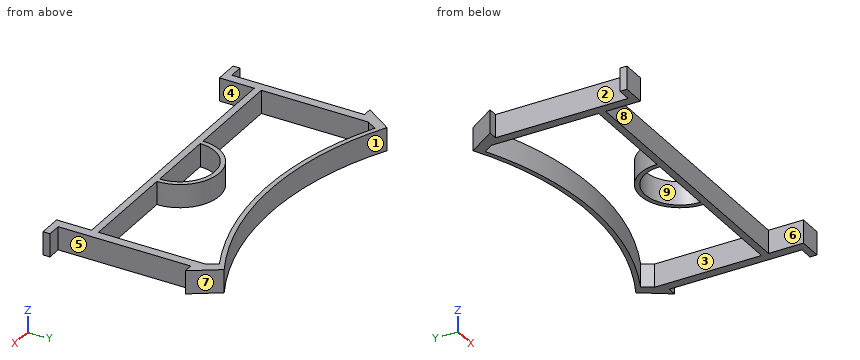
```python
from build123d import *

# Parameters (mm, degrees)
F1_DEPTH = 10


with BuildPart() as f1:
    # F0 (on Top) → F1 (new body)
    with BuildSketch(Plane.XY):
        with BuildLine():
            Line((0, 15), (0, 0))
            Line((0, 0), (10, 0))
            Line((10, 0), (10, 3))
            Line((10, 3), (4, 3))
            Line((4, 3), (4, 60))
            Line((4, 60), (8, 60))
            Line((8, 60), (0, 72))
            ThreePointArc((0, 72), (-60, 57.325626), (-120, 72))
            Line((-120, 72), (-128, 60))
            Line((-128, 60), (-124, 60))
            Line((-124, 60), (-124, 3))
            Line((-124, 3), (-130, 3))
            Line((-130, 3), (-130, 0))
            Line((-130, 0), (-120, 0))
            Line((-120, 0), (-120, 15))
            Line((-120, 15), (-120, 18))
            Line((-120, 18), (-120, 60))
            Line((-120, 60), (-120, 64))
            Line((-120, 64), (-117.309005, 68.39129))
            ThreePointArc((-117.309005, 68.39129), (-60, 55.232971), (-2.690995, 68.39129))
            Line((-2.690995, 68.39129), (0, 64))
            Line((0, 64), (0, 60))
            Line((0, 60), (0, 18))
            Line((0, 18), (0, 15))
        make_face()
        Polygon((-120, 15), (0, 15), (0, 18), (-43, 18), (-45, 18), (-75, 18), (-77, 18), (-120, 18), align=None)
        with BuildLine():
            Line((-45, 18), (-43, 18))
            ThreePointArc((-43, 18), (-60, 35), (-77, 18))
            Line((-77, 18), (-75, 18))
            ThreePointArc((-75, 18), (-60, 33), (-45, 18))
        make_face()
    extrude(amount=F1_DEPTH)


solid = f1.part
```
Verification items for the finished model (mm, model axes). Face numbers are marked on the shaded views. A direction names the side the tool comes from. Round coordinates to 2 decimals unless told otherwise and drop trailing zeros. Loops run counter-clockwise (first coordinate to the right, second up) from the corner with the lowest first, then second, coordinate; pieces in that order, holes last. Notation, with made-up numbers: (6.25, -34.5) -> (43.25, -34.5) arc R24 cw to (43.25, -4.5) -> close; hole circle Ø8 at (79, 15). An arc over 180 degrees is marked (long way). Answer as a JSON object with one key per item and string values.
Q1. Scan lines: line 1 (Y direction, x = -49, z = 3.25); line 2 (X direction, y = 10, z = 4.5); line 3 (Y direction, x = -68, z = 2). Record each from-to range of solid material in increasing order. Write a range as from..to.
Data:
{"line 1": "y = 15..18, 28.2..30.96, 55.69..57.79", "line 2": "x = -124..-120, 0..4", "line 3": "y = 15..18, 30.69..33, 55.48..57.57"}
Q2. Section check C-C (y = 50). Record the boundary of the cut face in (x, z).
Data:
{"outline": "(-124, 0) -> (-120, 0) -> (-120, 10) -> (-124, 10) -> close; (0, 0) -> (4, 0) -> (4, 10) -> (0, 10) -> close"}
Q3. Go/stop test with flat-tipped pins: P1, Ø3, axis at y = 40.5, z = 6.5, coming from the -X side; P2, Ø1.8, axis at x = 7.5, z = 5.5, coming from the +Y side; P3, Ø4, axis at y = 29.5, z = 2, coming from the +X side; P4, Ø10, axis at x = -85.5, y = 7.5, coming from the -Z side. Record where each tip stops, or that it passes through.
Data:
{"P1": "stops at x = -124", "P2": "stops at y = 62.1", "P3": "stops at x = 4", "P4": "passes through"}
Q4. Section check D-D (x = -31). Record the boundary of the cut face in (y, z), then the cut area to 3 significant figures.
Data:
{"outline": "(15, 0) -> (18, 0) -> (18, 10) -> (15, 10) -> close; (58.47, 0) -> (60.6, 0) -> (60.6, 10) -> (58.47, 10) -> close", "area": "51.3 mm2"}
Q5. Section check B-B (z = 2.25). Record the boundary of the cut face in (x, y), then the cut area to 3 significant figures.
Data:
{"outline": "(-130, 0) -> (-120, 0) -> (-120, 15) -> (0, 15) -> (0, 0) -> (10, 0) -> (10, 3) -> (4, 3) -> (4, 60) -> (8, 60) -> (0, 72) arc R130 cw to (-120, 72) -> (-128, 60) -> (-124, 60) -> (-124, 3) -> (-130, 3) -> close; hole (-120, 18) -> (-77, 18) arc R17 cw to (-43, 18) -> (0, 18) -> (0, 64) -> (-2.69, 68.39) arc R131.38 cw to (-117.31, 68.39) -> (-120, 64) -> close; hole (-75, 18) -> (-45, 18) arc R15 ccw to start", "area": "1,350 mm2"}
Q6. Draft check along Y on the marked faces 6, 7, 8 and 9. Enter one of: pulls with the +Y half, pulls with the -Y half, needs draft (parallel to the pull), parting line crosses it, or undercut.
Data:
{"face 6": "needs draft", "face 7": "pulls with the +Y half", "face 8": "pulls with the -Y half", "face 9": "undercut"}
Q7. Section check A-A (x = -60). Record the boundary of the cut face in (y, z), then the cut area to 3 significant figures.
Data:
{"outline": "(15, 0) -> (18, 0) -> (18, 10) -> (15, 10) -> close; (33, 0) -> (35, 0) -> (35, 10) -> (33, 10) -> close; (55.23, 0) -> (57.33, 0) -> (57.33, 10) -> (55.23, 10) -> close", "area": "70.9 mm2"}
Q8. Access from +Z, -Z, +X, -X, +Y, -Y to the whole of each face (thin tool, end or side, straight path). Record for the marked faces 1, 2, 3, 4 and 5.
Data:
{"face 1": "+Z, -Z, +Y", "face 2": "+Z, -Z, -X", "face 3": "+Z, -Z", "face 4": "+Z, -Z, -Y", "face 5": "+Z, -Z, +X"}
